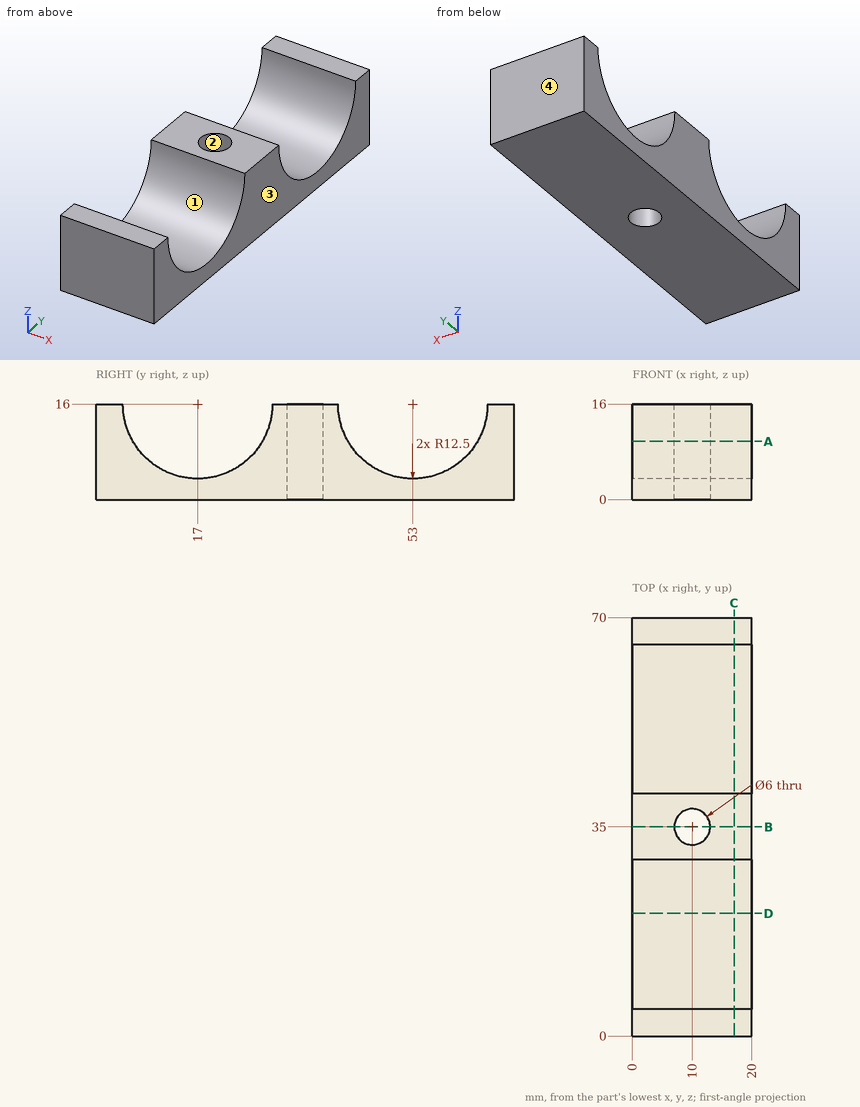
Source: three-view drawing plus pictorial views. Frame: mm from the lowest corner of the part. Coordinates: 2 decimals unless noted, no trailing zeros. Order: outer loops, then holes, each group sorted by start corner. A loop starts at its lowest first (then second) coordinate and runs counter-clockwise, first axis right, second up.
1) Section C-C (x = 17). Return loops of the section in (y, z).
Result sheet:
outline: (0, 0) - (70, 0) - (70, 16) - (65.5, 16) arc R12.5 cw to (40.5, 16) - (29.5, 16) arc R12.5 cw to (4.5, 16) - (0, 16) - close
2) Section A-A (z = 9.75). Return loops of the section in (x, y), then the cut area to 3 significant figures.
Result sheet:
outline: (0, 0) - (20, 0) - (20, 6.17) - (0, 6.17) - close; (0, 27.83) - (20, 27.83) - (20, 42.17) - (0, 42.17) - close; (0, 63.83) - (20, 63.83) - (20, 70) - (0, 70) - close; hole circle Ø6 at (10, 35)
area: 506 mm2
3) Draft query along Y for the marked faces 1, 2, 3 and 4. Return one class per face: released by +Y, released by -Y, zero draft, split by the parting line, or undercut.
Result sheet:
face 1: undercut
face 2: undercut
face 3: zero draft
face 4: released by +Y
4) Section D-D (y = 20.5). Return loops of the section in (x, z).
Result sheet:
outline: (0, 0) - (20, 0) - (20, 4) - (0, 4) - close
5) Section B-B (y = 35). Return loops of the section in (x, z).
Result sheet:
outline: (0, 0) - (7, 0) - (7, 16) - (0, 16) - close; (13, 0) - (20, 0) - (20, 16) - (13, 16) - close
6) Ray query, probe 1 along Y at (x, z) = (18, 15); probe 2 along Y at (x, z) = (13.25, 8); probe 3 along Y at (x, z) = (10, 9.25). Return the intervals inside material, ascending.
Result sheet:
probe 1: y = 0 to 4.54, 29.46 to 40.54, 65.46 to 70
probe 2: y = 0 to 7.4, 26.6 to 43.4, 62.6 to 70
probe 3: y = 0 to 6.48, 27.52 to 32, 38 to 42.48, 63.52 to 70
7) First-contact query: P1, Ø4, axis at x = 5.5, y = 49, coming from the +Z side; P2, Ø4, axis at x = 7.5, y = 13.5, coming from the +Z side (3 decimals); P3, Ø4, axis at x = 6, y = 54, coming from the +Z side; P4, Ø5, axis at x = 10, y = 35, coming from the -Z side. Flat tips, straight axial feed; report the tip coordinate or a pass-through.
Result sheet:
P1: stops at z = 5.03
P2: stops at z = 4.775
P3: stops at z = 3.87
P4: passes through
